Input: part model. Units: mm. Frame: model coordinates. Give positions to 0.01 mm unless a question says otherwise; leave off trailing zeros. Write each loop counter-clockwise with the first axis right and the second up, starting at its lowest first coordinate (ties: lowest second). Pieces come first, ordered by that corner, then holes. Notation, with made-up numbers: (-17, 71) - (35, 71) arc R23 cw to (35, 100) - close; hole circle Ø1 at (-0.75, 8.5). An arc over 180 degrees is marked (long way). Answer as CSV lines item,"result".
```python
from build123d import *

# Parameters (mm, degrees)
Y_KSEKLIK_EKSTR_ZYON1_DEPTH = 2
IZIM2_R                     = 9
KES_EKSTR_ZYON1_DEPTH       = 5


with BuildPart() as part:
    # Çizim1 → Yükseklik-Ekstrüzyon1 (new body, symmetric)
    with BuildSketch(Plane.XY):
        with BuildLine():
            Line((0, 0), (0, 110))
            Line((0, 110), (32, 110))
            Line((32, 110), (32, 85))
            ThreePointArc((32, 85), (22.190316578, 48.5), (32, 12))
            Line((32, 12), (32, 0))
            Line((32, 0), (0, 0))
        make_face()
    extrude(amount=Y_KSEKLIK_EKSTR_ZYON1_DEPTH, both=True)

    # Çizim2 → Kes-Ekstrüzyon1 (cut, through all)
    with BuildSketch(Plane.XY.offset(2)):
        with Locations((13, 93.5)):
            Circle(IZIM2_R)
        with Locations((13, 18.5)):
            Circle(IZIM2_R)
    extrude(amount=-KES_EKSTR_ZYON1_DEPTH, mode=Mode.SUBTRACT)


solid = part.part
```
Item 1: Mould query, pull axis X, two halves, no side actions, for faces 1 (the face through (11.828, 27.423, 0.028)), 2 (the face through (13, 56, 2)), 3 (the face through (0, 54, 0)). Classes: +X half, -X half, draft (parallel to the pull), parting line (faces both ways), or undercut.
The answers:
face 1,"undercut"
face 2,"draft"
face 3,"-X half"
Item 2: Cut plane A-A on x = 13. Return the cut outline in (y, z), plus the area to 3 significant figures.
The answers:
outline,"(0, -2) - (9.5, -2) - (9.5, 2) - (0, 2) - close; (27.5, -2) - (84.5, -2) - (84.5, 2) - (27.5, 2) - close; (102.5, -2) - (110, -2) - (110, 2) - (102.5, 2) - close"
area,"296 mm²"
Item 3: Cut plane D-D on x = 29. Return the cut outline in (y, z), plus the area to 3 significant figures.
The answers:
outline,"(0, -2) - (17.76, -2) - (17.76, 2) - (0, 2) - close; (79.24, -2) - (110, -2) - (110, 2) - (79.24, 2) - close"
area,"194 mm²"
Item 4: Contact query for flat-ended pins moving along their axis: pin 1 (1 mm diameter, centred on y = 33, z = 1, fed in from +X); pin 2 (2 mm diameter, centred on y = 25.5, z = 1, fed in from +X); pin 3 (1.5 mm diameter, centred on x = 25.5, z = -0.5, fed in from -Y). Output: stop coordinate, or through.
The answers:
pin 1,"x = 23.97"
pin 2,"x = 26.26"
pin 3,"y = 0"
Item 5: Cut plane B-B on z = 1.2. Return the cut outline in (x, y), plus the area to 3 significant figures.
The answers:
outline,"(0, 0) - (32, 0) - (32, 12) arc R72.81 cw to (32, 85) - (32, 110) - (0, 110) - close; hole circle Ø18 at (13, 18.5); hole circle Ø18 at (13, 93.5)"
area,"2,530 mm²"
Item 6: Cut plane C-C on y = 93.5. Return the cut outline in (x, z), plus the area to 3 significant figures.
The answers:
outline,"(0, -2) - (4, -2) - (4, 2) - (0, 2) - close; (22, -2) - (32, -2) - (32, 2) - (22, 2) - close"
area,"56.0 mm²"
Item 7: Ray query, line 1 (Y direction, x = 13, z = -0.75); line 2 (X direction, y = 94, z = 1.55); line 3 (Y direction, x = 7.5, z = 1.4). Return the intervals inside material, ascending. Write a range as from..to.
The answers:
line 1,"0..9.5, 27.5..84.5, 102.5..110"
line 2,"0..4.01, 21.99..32"
line 3,"0..11.38, 25.62..86.38, 100.62..110"
